Geometry check sheet. Reference: the model listing, model coordinates, mm. Give positions to 0.01 mm unless a question says otherwise; leave off trailing zeros. Write each loop counter-clockwise with the first axis right and the second up, starting at its lowest first coordinate (ties: lowest second). Pieces come first, ordered by that corner, then holes. Notation, with made-up numbers: (81.25, 71.5) - (132.25, 71.5) arc R16 cw to (132.25, 85.5) - close; hole circle Ø8 at (75.5, -10.5). An arc over 180 degrees is marked (long way). One line per question, with ' | ' between items. Start each with the question number.
Q1. Thickness scan on L1, parallel to X at y = -7, z = 0; L2, parallel to X at y = 4.5, z = 0; L3, parallel to Z at x = -2, y = 7. Record the ranges inside material, lowest first. Write a range as [from, to].
Q2. Section check A-A on y = -5. Record the boundary of the cut face in (x, z).
Q3. Section check B-B on y = -15. Record the boundary of the cut face in (x, z), and give its area (3 significant figures).
Q4. Gauge pin test, flat ends, axial feed: P1, Ø5, axis at y = -15.5, z = -13.5, coming from the +X side; P2, Ø3, axis at y = 3.5, z = -9.5, coming from the +X side; P3, Ø3, axis at y = -6, z = -5, coming from the +X side. Record the tip position at first contact, or that the pin passes through.
```python
from build123d import *

# Parameters (mm, degrees)
CHAMFER_1_SIZE = 0.5


with BuildPart() as part:
    # Sketch 1 → Revolve 1 (revolve)
    with BuildSketch(Plane.XY, mode=Mode.PRIVATE) as revolve_1_sk:
        Polygon((7, 22.5), (17.5, 22.5), (17.5, 10.5), (17.2, 10.5), (17.2, 9), (17.5, 9), (17.5, 5.625), (17.2, 5.625), (17.2, 4.125), (17.5, 4.125), (17.5, 0.75), (17.2, 0.75), (17.2, -0.75), (17.5, -0.75), (17.5, -4.125), (17.2, -4.125), (17.2, -5.625), (17.5, -5.625), (17.5, -9), (17.2, -9), (17.2, -10.5), (17.5, -10.5), (17.5, -22.5), (7, -22.5), align=None)
    revolve(revolve_1_sk.sketch.rotate(Axis((0, 53.65103478, 0), (0, -1, 0)), 90), axis=Axis((0, 53.65103478, 0), (0, -1, 0)))

    # Chamfer 1
    chamfer_1_edges = [part.edges().sort_by_distance(p)[0] for p in [
        (0, 22.5, -7),
        (0, 22.5, -17.5),
        (0, -22.5, -17.5),
        (0, -22.5, -7),
    ]]
    chamfer(chamfer_1_edges, length=CHAMFER_1_SIZE)


solid = part.part
```
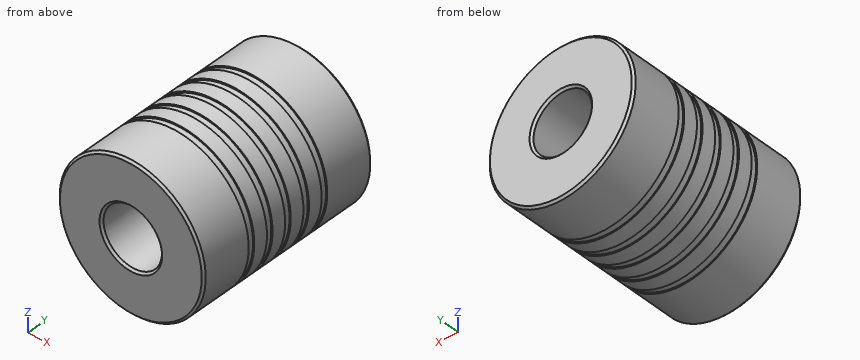
Working result:
1) L1: x = [-17.5, -7], [7, 17.5] | L2: x = [-17.2, -7], [7, 17.2] | L3: z = [-17.39, -6.71], [6.71, 17.39]
2) outline: circle Ø34.4 at (0, 0); hole circle Ø14 at (0, 0)
3) outline: circle Ø35 at (0, 0); hole circle Ø14 at (0, 0) | area: 808 mm2
4) P1: stops at x = 13.61 | P2: stops at x = 15.56 | P3: stops at x = 17.15
